CAD build for the part. Positions are in the model's coordinates, mm. Face numbers are marked on the shaded views. A direction names the side the tool comes from. Coordinates: 2 decimals unless noted, no trailing zeros. Order: outer loops, then holes, each group sorted by start corner. A loop starts at its lowest first (then second) coordinate and runs counter-clockwise, first axis right, second up. Notation, with made-up numbers: M 65.25,-4 L 89.25,-4 A14 ccw 89.25,21 Z; hole C 51,66.25 d3. An arc over 180 degrees is marked long. Write item = value, one per line.
from build123d import *

# Parameters (mm, degrees)
SKETCH_1_W           = 46
SKETCH_1_H           = 34
EXTRUDE_1_DEPTH      = 7
CUT_EXTRUDE_1_DEPTH  = 1.6
CUT_EXTRUDE_2_DEPTH  = 3.5
FILLET_1_R           = 1
FILLET_2_R           = 4
SKETCH_5_R           = 0.85
CUT_EXTRUDE_3_DEPTH  = 4
CUT_EXTRUDE_4_REACH  = 51.538
CUT_EXTRUDE_5_DEPTH  = 2
SKETCH_7_W           = 9.4
SKETCH_7_H           = 3
CUT_EXTRUDE_6_DEPTH  = 3
SKETCH_8_W           = 11.4
SKETCH_8_H           = 5
SKETCH_8_W_2         = 9.4
SKETCH_8_H_2         = 3
CUT_EXTRUDE_7_DEPTH  = 2
FILLET_3_R           = 1
EXTRUDE_START        = 3.5
EXTRUDE_2_DEPTH      = 3.5
CHAMFER_1_SIZE       = 1
CUT_EXTRUDE_9_DEPTH  = 1.6
CUT_EXTRUDE_10_REACH = 31.106
SKETCH_11_W          = 0.5
SKETCH_11_H          = 8.840000414
CUT_EXTRUDE_11_DEPTH = 2


with BuildPart() as part:
    # 草图1 → 凸台-拉伸1 (new body)
    with BuildSketch(Plane.XY):
        Rectangle(SKETCH_1_W, SKETCH_1_H)
    extrude(amount=EXTRUDE_1_DEPTH)

    # 草图3 → 切除-拉伸1 (cut)
    with BuildSketch(Plane.XY.offset(7)):
        with BuildLine():
            Line((-18, -14), (18, -14))
            ThreePointArc((18, -14), (19.414213562, -13.414213562), (20, -12))
            Line((20, -12), (20, 12))
            ThreePointArc((20, 12), (19.414213562, 13.414213562), (18, 14))
            Line((18, 14), (-18, 14))
            ThreePointArc((-18, 14), (-19.414213562, 13.414213562), (-20, 12))
            Line((-20, 12), (-20, -12))
            ThreePointArc((-20, -12), (-19.414213562, -13.414213562), (-18, -14))
        make_face()
    extrude(amount=-CUT_EXTRUDE_1_DEPTH, mode=Mode.SUBTRACT)

    # 草图4 → 切除-拉伸2 (cut)
    with BuildSketch(Plane.XY.offset(5.4)):
        with BuildLine():
            ThreePointArc((20, 12), (16.585786438, 10.585786438), (18, 14))
            Line((18, 14), (-18, 14))
            ThreePointArc((-18, 14), (-16.585786438, 13.414213562), (-16, 12))
            ThreePointArc((-16, 12), (-18, 10), (-20, 12))
            Line((-20, 12), (-20, -12))
            ThreePointArc((-20, -12), (-19.414213562, -13.414213562), (-18, -14))
            Line((-18, -14), (18, -14))
            ThreePointArc((18, -14), (16.585786438, -10.585786438), (20, -12))
            Line((20, -12), (20, 12))
        make_face()
    extrude(amount=-CUT_EXTRUDE_2_DEPTH, mode=Mode.SUBTRACT)

    # 圆角1
    fillet_1_edges = [part.edges().sort_by_distance(p)[0] for p in [
        (18, 14, 3.65),
        (20, 12, 3.65),
        (20, -12, 3.65),
        (18, -14, 3.65),
        (-20, 12, 3.65),
        (-18, 14, 3.65),
    ]]
    fillet(fillet_1_edges, radius=FILLET_1_R)

    # 圆角2
    fillet_2_edges = [part.edges().sort_by_distance(p)[0] for p in [
        (23, -17, 3.5),
        (-23, -17, 3.5),
        (-23, 17, 3.5),
        (23, 17, 3.5),
    ]]
    fillet(fillet_2_edges, radius=FILLET_2_R)

    # 草图5 → 切除-拉伸3 (cut)
    with BuildSketch(Plane.XY.offset(5.4)):
        with Locations((-18, 12)):
            Circle(SKETCH_5_R)
        with Locations((18, 12)):
            Circle(SKETCH_5_R)
        with Locations((18, -12)):
            Circle(SKETCH_5_R)
    extrude(amount=-CUT_EXTRUDE_3_DEPTH, mode=Mode.SUBTRACT)

    # 草图6 → 切除-拉伸4 (cut, up to next)
    with BuildSketch(Plane.ZY.offset(23), mode=Mode.PRIVATE) as cut_extrude_4_sk1:
        with BuildLine():
            Line((4.109999831, 6.325004017), (3.349999795, 6.325004017))
            ThreePointArc((3.349999795, 6.325004017), (2.536826958, 5.9881768), (2.199999741, 5.175003963))
            Line((2.199999741, 5.175003963), (2.199999741, -1.364996343))
            ThreePointArc((2.199999741, -1.364996343), (2.536826958, -2.17816918), (3.349999795, -2.514996397))
            Line((3.349999795, -2.514996397), (4.109999831, -2.514996397))
            ThreePointArc((4.109999831, -2.514996397), (4.923172667, -2.17816918), (5.259999885, -1.364996343))
            Line((5.259999885, -1.364996343), (5.259999885, 5.175003963))
            ThreePointArc((5.259999885, 5.175003963), (4.923172667, 5.9881768), (4.109999831, 6.325004017))
        make_face()
    cut_extrude_4_tool1 = extrude(cut_extrude_4_sk1.sketch, amount=-CUT_EXTRUDE_4_REACH, mode=Mode.PRIVATE) & part.part
    add(cut_extrude_4_tool1.solids().sort_by_distance((-23, 1.905004, 3.73))[0], mode=Mode.SUBTRACT)

    # 草图6<3> → 切除-拉伸5 (cut)
    with BuildSketch(Plane.ZY.offset(23)):
        with BuildLine():
            Line((3.349999795, -4.014996397), (4.109999831, -4.014996397))
            ThreePointArc((4.109999831, -4.014996397), (5.983832839, -3.238829352), (6.759999885, -1.364996343))
            Line((6.759999885, -1.364996343), (6.759999885, 5.175003963))
            ThreePointArc((6.759999885, 5.175003963), (5.983832839, 7.048836972), (4.109999831, 7.825004017))
            Line((4.109999831, 7.825004017), (3.349999795, 7.825004017))
            ThreePointArc((3.349999795, 7.825004017), (1.476166787, 7.048836972), (0.699999741, 5.175003963))
            Line((0.699999741, 5.175003963), (0.699999741, -1.364996343))
            ThreePointArc((0.699999741, -1.364996343), (1.476166787, -3.238829352), (3.349999795, -4.014996397))
        make_face()
        with BuildLine():
            Line((3.349999795, -2.514996397), (4.109999831, -2.514996397))
            ThreePointArc((4.109999831, -2.514996397), (4.923172667, -2.17816918), (5.259999885, -1.364996343))
            Line((5.259999885, -1.364996343), (5.259999885, 5.175003963))
            ThreePointArc((5.259999885, 5.175003963), (4.923172667, 5.9881768), (4.109999831, 6.325004017))
            Line((4.109999831, 6.325004017), (3.349999795, 6.325004017))
            ThreePointArc((3.349999795, 6.325004017), (2.536826958, 5.9881768), (2.199999741, 5.175003963))
            Line((2.199999741, 5.175003963), (2.199999741, -1.364996343))
            ThreePointArc((2.199999741, -1.364996343), (2.536826958, -2.17816918), (3.349999795, -2.514996397))
        make_face(mode=Mode.SUBTRACT)
    extrude(amount=-CUT_EXTRUDE_5_DEPTH, mode=Mode.SUBTRACT)

    # 草图7 → 切除-拉伸6 (cut)
    with BuildSketch(Plane.XZ.offset(17)):
        with Locations((0, 3.4)):
            Rectangle(SKETCH_7_W, SKETCH_7_H)
    extrude(amount=-CUT_EXTRUDE_6_DEPTH, mode=Mode.SUBTRACT)

    # 草图8 → 切除-拉伸7 (cut)
    with BuildSketch(Plane.XZ.offset(17)):
        with Locations((0, 3.4)):
            Rectangle(SKETCH_8_W, SKETCH_8_H)
        with Locations((0, 3.4)):
            Rectangle(SKETCH_8_W_2, SKETCH_8_H_2, mode=Mode.SUBTRACT)
    extrude(amount=-CUT_EXTRUDE_7_DEPTH, mode=Mode.SUBTRACT)

    # 圆角3
    fillet_3_edges = [part.edges().sort_by_distance(p)[0] for p in [
        (5.7, -16, 0.9),
        (-5.7, -16, 0.9),
        (-5.7, -16, 5.9),
        (5.7, -16, 5.9),
    ]]
    fillet(fillet_3_edges, radius=FILLET_3_R)

    # 草图9 → 凸台-拉伸2 (add)
    with BuildSketch(Plane.XY.offset(7).offset(EXTRUDE_START)):
        with BuildLine():
            Line((-19, -17), (19, -17))
            ThreePointArc((19, -17), (21.828427125, -15.828427125), (23, -13))
            Line((23, -13), (23, 13))
            ThreePointArc((23, 13), (21.828427125, 15.828427125), (19, 17))
            Line((19, 17), (-19, 17))
            ThreePointArc((-19, 17), (-21.828427125, 15.828427125), (-23, 13))
            Line((-23, 13), (-23, -13))
            ThreePointArc((-23, -13), (-21.828427125, -15.828427125), (-19, -17))
        make_face()
        with BuildLine():
            Line((-19, -15), (19, -15))
            ThreePointArc((19, -15), (20.414213562, -14.414213562), (21, -13))
            Line((21, -13), (21, 13))
            ThreePointArc((21, 13), (20.414213562, 14.414213562), (19, 15))
            Line((19, 15), (-19, 15))
            ThreePointArc((-19, 15), (-20.414213562, 14.414213562), (-21, 13))
            Line((-21, 13), (-21, -13))
            ThreePointArc((-21, -13), (-20.414213562, -14.414213562), (-19, -15))
        make_face(mode=Mode.SUBTRACT)
    extrude(amount=-EXTRUDE_2_DEPTH)

    # 倒角1
    # the kernel refuses this chamfer: 1 mm, written as the material it takes off along each edge
    with BuildSketch(Plane(origin=(19, 13, 0), x_dir=(1, 0, 0), z_dir=(0, -1, 0))) as chamfer_1_piece_1:
        Polygon((4, CHAMFER_1_SIZE), (4 - CHAMFER_1_SIZE, 0), (4, 0), align=None)
    revolve(axis=Axis((19, 13, 0), (0, 0, 1)), revolution_arc=90, mode=Mode.SUBTRACT)
    with BuildSketch(Plane(origin=(19, 17, 0), x_dir=(0, 0.02749587661058563, 0.9996219169112968), z_dir=(-1, 0, 0)), Plane(origin=(-19, -17, 0), x_dir=(0, -0.02749587661058563, 0.9996219169112968), z_dir=(1, 0, 0))) as chamfer_1_piece_2:
        Polygon((CHAMFER_1_SIZE * 0.999621916911, -CHAMFER_1_SIZE * 0.0274958766106), (-CHAMFER_1_SIZE * 0.0274958766106, -CHAMFER_1_SIZE * 0.999621916911), (0, 0), align=None)
    extrude(amount=38, mode=Mode.SUBTRACT)
    with BuildSketch(Plane(origin=(-19, 13, 0), x_dir=(-1, 0, 0), z_dir=(0, -1, 0))) as chamfer_1_piece_3:
        Polygon((4, -CHAMFER_1_SIZE), (4 - CHAMFER_1_SIZE, 0), (4, 0), align=None)
    revolve(axis=Axis((-19, 13, 0), (0, 0, -1)), revolution_arc=90, mode=Mode.SUBTRACT)
    with BuildSketch(Plane(origin=(-23, 13, 0), x_dir=(-0.02749587661058563, 0, 0.9996219169112968), z_dir=(0, -1, 0)), Plane(origin=(23, -13, 0), x_dir=(0.02749587661058563, 0, 0.9996219169112968), z_dir=(0, 1, 0))) as chamfer_1_piece_4:
        Polygon((CHAMFER_1_SIZE * 0.999621916911, -CHAMFER_1_SIZE * 0.0274958766106), (-CHAMFER_1_SIZE * 0.0274958766106, -CHAMFER_1_SIZE * 0.999621916911), (0, 0), align=None)
    extrude(amount=26, mode=Mode.SUBTRACT)
    with BuildSketch(Plane(origin=(-19, -13, 0), x_dir=(0, -1, 0), z_dir=(1, 0, 0))) as chamfer_1_piece_5:
        Polygon((4, -CHAMFER_1_SIZE), (4 - CHAMFER_1_SIZE, 0), (4, 0), align=None)
    revolve(axis=Axis((-19, -13, 0), (0, 0, -1)), revolution_arc=90, mode=Mode.SUBTRACT)
    with BuildSketch(Plane(origin=(19, -13, 0), x_dir=(0, -1, 0), z_dir=(-1, 0, 0))) as chamfer_1_piece_6:
        Polygon((4, CHAMFER_1_SIZE), (4 - CHAMFER_1_SIZE, 0), (4, 0), align=None)
    revolve(axis=Axis((19, -13, 0), (0, 0, 1)), revolution_arc=90, mode=Mode.SUBTRACT)

    # 草图10 → 切除-拉伸9 (cut)
    # profile 1 of 2: a face of its own
    with BuildSketch(Plane.XY.offset(7)):
        with BuildLine():
            Line((-18, -14.5), (18, -14.5))
            ThreePointArc((18, -14.5), (19.767766953, -13.767766953), (20.5, -12))
            Line((20.5, -12), (20.5, 12))
            ThreePointArc((20.5, 12), (19.767766953, 13.767766953), (18, 14.5))
            Line((18, 14.5), (-18, 14.5))
            ThreePointArc((-18, 14.5), (-19.767766953, 13.767766953), (-20.5, 12))
            Line((-20.5, 12), (-20.5, 9.171572875))
            Line((-20.5, 9.171572875), (-20.5, -12))
            ThreePointArc((-20.5, -12), (-19.767766953, -13.767766953), (-18, -14.5))
        make_face()
        with BuildLine():
            ThreePointArc((-20, 12), (-19.414213562, 13.414213562), (-18, 14))
            Line((-18, 14), (18, 14))
            ThreePointArc((18, 14), (19.414213562, 13.414213562), (20, 12))
            Line((20, 12), (20, -12))
            ThreePointArc((20, -12), (19.414213562, -13.414213562), (18, -14))
            Line((18, -14), (-18, -14))
            ThreePointArc((-18, -14), (-19.414213562, -13.414213562), (-20, -12))
            Line((-20, -12), (-20, 12))
        make_face(mode=Mode.SUBTRACT)
    # profile 2 of 2: a face of its own
    with BuildSketch(Plane.XY.offset(7)):
        with BuildLine():
            ThreePointArc((20, 12), (19.414213562, 13.414213562), (18, 14))
            Line((18, 14), (-18, 14))
            ThreePointArc((-18, 14), (-19.414213562, 13.414213562), (-20, 12))
            Line((-20, 12), (-20, 9.171572875))
            Line((-20, 9.171572875), (-20, -12))
            ThreePointArc((-20, -12), (-19.414213562, -13.414213562), (-18, -14))
            Line((-18, -14), (18, -14))
            ThreePointArc((18, -14), (19.414213562, -13.414213562), (20, -12))
            Line((20, -12), (20, 12))
        make_face()
    extrude(amount=-CUT_EXTRUDE_9_DEPTH, mode=Mode.SUBTRACT)

    # 草图11 → 切除-拉伸10 (cut, up to next)
    with BuildSketch(Plane.XY.offset(5.4), mode=Mode.PRIVATE) as cut_extrude_10_sk1:
        with Locations((-20.25, 1.90500381)):
            Rectangle(SKETCH_11_W, SKETCH_11_H)
    cut_extrude_10_tool1 = extrude(cut_extrude_10_sk1.sketch, amount=-CUT_EXTRUDE_10_REACH, mode=Mode.PRIVATE) & part.part
    add(cut_extrude_10_tool1.solids().sort_by_distance((-20.25, 1.905004, 5.4))[0], mode=Mode.SUBTRACT)

    # 草图12 → 切除-拉伸11 (cut)
    with BuildSketch(Plane.ZY.offset(23)):
        with BuildLine():
            Line((0.599999741, 5.175003963), (0.599999741, -1.364996343))
            ThreePointArc((0.599999741, -1.364996343), (1.405456108, -3.30954003), (3.349999795, -4.114996397))
            Line((3.349999795, -4.114996397), (4.109999831, -4.114996397))
            ThreePointArc((4.109999831, -4.114996397), (6.054543517, -3.30954003), (6.859999885, -1.364996343))
            Line((6.859999885, -1.364996343), (6.859999885, 5.175003963))
            ThreePointArc((6.859999885, 5.175003963), (6.054543517, 7.11954765), (4.109999831, 7.925004017))
            Line((4.109999831, 7.925004017), (3.349999795, 7.925004017))
            ThreePointArc((3.349999795, 7.925004017), (1.405456108, 7.11954765), (0.599999741, 5.175003963))
        make_face()
    extrude(amount=-CUT_EXTRUDE_11_DEPTH, mode=Mode.SUBTRACT)


solid = part.part
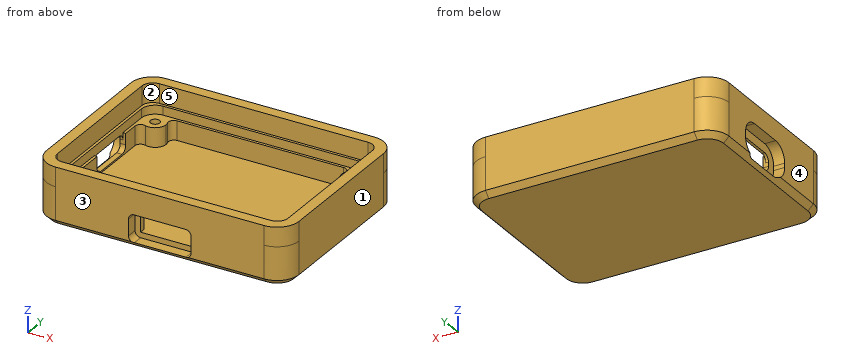
(1) Slice it at C-C, the plane y = 8.5. Write the cut outline in (x, z), then the cut area to 3 significant figures.
Evaluation:
outline = M -23,1 L -22,0 L 22,0 L 23,1 L 23,10.5 L 21,10.5 L 21,7 L 20.5,7 L 20.5,5.4 L 20,5.4 L 20,1.9 L -20,1.9 L -20,5.4 L -20.5,5.4 L -20.5,7 L -21,7 L -21,10.5 L -23,10.5 Z
area = 129 mm²
(2) Tool access for the marked faces 1 and 2: list every direction of +Z, -Z, +X, -X, +Y, -Y with a clear straight run to the whole face (end or side of a thin tool).
Evaluation:
face_1 = +Z, -Z, +X, +Y, -Y
face_2 = +Z
(3) Wall check: line 1 (Y direction, x = 18, z = 4.35); line 2 (Y direction, x = -18, z = 3.35); line 3 (X direction, y = 4.5, z = 7.5). Give the ranges that are in metal, low to high. Write a range as from..to.
Evaluation:
line_1 = -17..-12.85, -11.15..-10, 10..11.15, 12.85..17
line_2 = -17..-14, 10..11.15, 12.85..17
line_3 = -23..-21, 21..23
(4) Pull direction Y, two halves, no side cores. Call the marked faces 3, 4 and 5: +Y half, -Y half, draft (parallel to the pull), parting line (faces both ways), or undercut.
Evaluation:
face_3 = -Y half
face_4 = draft
face_5 = undercut
(5) Slice it at B-B, the plane x = 1.5. Write the cut outline in (y, z), then the cut area to 3 significant figures.
Evaluation:
outline = M -17,5.9 L -15,5.9 L -15,4.9 L -14,4.9 L -14,5.4 L -14.5,5.4 L -14.5,7 L -15,7 L -15,10.5 L -17,10.5 Z; M -16.9,0.9 L -16,0 L 16,0 L 17,1 L 17,10.5 L 15,10.5 L 15,7 L 14.5,7 L 14.5,5.4 L 14,5.4 L 14,1.9 L -15,1.9 L -15,0.9 Z
area = 93.6 mm²
(6) Slice it at A-A, the plane z = 8. Write the cut outline in (x, y).
Evaluation:
outline = M -23,-13 A4 ccw -19,-17 L 19,-17 A4 ccw 23,-13 L 23,13 A4 ccw 19,17 L -19,17 A4 ccw -23,13 Z; hole M -21,-13 A2 ccw -19,-15 L 19,-15 A2 ccw 21,-13 L 21,13 A2 ccw 19,15 L -19,15 A2 ccw -21,13 Z
(7) Pin check, flat tips, straight feed: pin 1 Ø3 at (y, z) = (3.5, 4) entering from -X; pin 2 Ø0.5 at (x, z) = (-20.5, 4.5) entering from -Y; pin 3 Ø0.6 at (y, z) = (-16.5, 3) entering from -X. Stop position of each tip, or through.
Evaluation:
pin_1 = -21
pin_2 = -16.8
pin_3 = -21.4
(8) Slice it at D-D, the plane x = -11.5. Write the cut outline in (y, z).
Evaluation:
outline = M -17,1 L -16,0 L 16,0 L 17,1 L 17,10.5 L 15,10.5 L 15,7 L 14.5,7 L 14.5,5.4 L 14,5.4 L 14,1.9 L -14,1.9 L -14,5.4 L -14.5,5.4 L -14.5,7 L -15,7 L -15,10.5 L -17,10.5 Z
